from build123d import *

# Parameters (mm, degrees)
SKETCH1_W               = 24
SKETCH1_H               = 21
SKETCH1_R               = 1.625
BOSS_EXTRUDE1_DEPTH     = 8
BOSS_EXTRUDE4_DEPTH     = 45
CUT_EXTRUDE9_DEPTH      = 57.756194596
CUT_EXTRUDE9_DEPTH_BACK = 57.756194596
SKETCH15_R              = 1.75
FILLET3_R               = 2.5
SKETCH4_R               = 2.5625
CUT_EXTRUDE3_DEPTH      = 3
FILLET7_R               = 0.5
SKETCH20_R              = 2.75
CUT_EXTRUDE15_DEPTH     = 4
CUT_EXTRUDE16_DEPTH     = 4


with BuildPart() as part:
    # Sketch1 → Boss-Extrude1 (new body)
    with BuildSketch(Plane(origin=(0, 0, 0), x_dir=(1, 0, 0), z_dir=(0, 1, 0))):
        Rectangle(SKETCH1_W, SKETCH1_H)
        with Locations(Location((-9.5, 8, 0), (0, 0, 270))):
            Circle(SKETCH1_R, mode=Mode.SUBTRACT)
        with Locations(Location((9.5, 8, 0), (0, 0, 270))):
            Circle(SKETCH1_R, mode=Mode.SUBTRACT)
        with Locations(Location((9.5, -8, 0), (0, 0, 270))):
            Circle(SKETCH1_R, mode=Mode.SUBTRACT)
        with Locations(Location((-9.5, -8, 0), (0, 0, 270))):
            Circle(SKETCH1_R, mode=Mode.SUBTRACT)
    extrude(amount=BOSS_EXTRUDE1_DEPTH)

    # Sketch7 → Boss-Extrude4 (add)
    with BuildSketch(Plane(origin=(12, 0, 0), x_dir=(0, 0, -1), z_dir=(1, 0, 0))):
        Polygon((-20.5625, 21), (-20.5625, 8), (20.5625, 8), (20.5625, 21), (15.0625, 21), (15.0625, 11), (-15.0625, 11), (-15.0625, 21), align=None)
    extrude(amount=-BOSS_EXTRUDE4_DEPTH)

    # Sketch15 → Cut-Extrude9 (cut, two sides: drawn at the far end of the back side and taken through both)
    with BuildSketch(Plane.XY.offset(20.5625).offset(-CUT_EXTRUDE9_DEPTH_BACK)):
        with Locations((7, 16)):
            Circle(SKETCH15_R)
        with Locations((-10.5, 16)):
            Circle(SKETCH15_R)
        with Locations((-28, 16)):
            Circle(SKETCH15_R)
    extrude(amount=CUT_EXTRUDE9_DEPTH + CUT_EXTRUDE9_DEPTH_BACK, mode=Mode.SUBTRACT)

    # Fillet3
    fillet3_edges = [part.edges().sort_by_distance(p)[0] for p in [
        (0, 8, -10.5),
        (-10.5, 8, -20.5625),
        (-10.5, 8, 20.5625),
        (-10.5, 21, 20.5625),
        (-10.5, 21, -20.5625),
        (-12, 8, 0),
        (0, 8, 10.5),
    ]]
    fillet(fillet3_edges, radius=FILLET3_R)

    # Sketch4 → Cut-Extrude3 (cut)
    with BuildSketch(Plane(origin=(0, 11, 0), x_dir=(1, 0, 0), z_dir=(0, 1, 0))):
        with Locations(Location((-9.5, 8, 0), (0, 0, 270))):
            Circle(SKETCH4_R)
        with Locations((9.5, 8)):
            Circle(SKETCH4_R)
        with Locations((9.5, -8)):
            Circle(SKETCH4_R)
        with Locations(Location((-9.5, -8, 0), (0, 0, 270))):
            Circle(SKETCH4_R)
    extrude(amount=-CUT_EXTRUDE3_DEPTH, mode=Mode.SUBTRACT)

    # Fillet7
    fillet7_edges = [part.edges().sort_by_distance(p)[0] for p in [
        (12, 9.5, 8.5625),
        (12, 9.5, 7.4375),
        (12, 9.5, -7.4375),
        (12, 9.5, -8.5625),
    ]]
    fillet(fillet7_edges, radius=FILLET7_R)

    # Sketch20 → Cut-Extrude15 (cut)
    with BuildSketch(Plane.XY.offset(20.5625)):
        with Locations((-28, 16)):
            Circle(SKETCH20_R)
        with Locations((-10.5, 16)):
            Circle(SKETCH20_R)
        with Locations((7, 16)):
            Circle(SKETCH20_R)
    extrude(amount=-CUT_EXTRUDE15_DEPTH, mode=Mode.SUBTRACT)

    # Sketch21 → Cut-Extrude16 (cut)
    with BuildSketch(Plane(origin=(0, 0, -20.5625), x_dir=(-1, 0, 0), z_dir=(0, 0, -1))):
        Polygon((-5.441154273, 13.3), (-3.882308546, 16), (-5.441154273, 18.7), (-8.558845727, 18.7), (-10.117691454, 16), (-8.558845727, 13.3), align=None)
        Polygon((12.058845727, 13.3), (13.617691454, 16), (12.058845727, 18.7), (8.941154273, 18.7), (7.382308546, 16), (8.941154273, 13.3), align=None)
        Polygon((29.558845727, 13.3), (31.117691454, 16), (29.558845727, 18.7), (26.441154273, 18.7), (24.882308546, 16), (26.441154273, 13.3), align=None)
    extrude(amount=-CUT_EXTRUDE16_DEPTH, mode=Mode.SUBTRACT)


solid = part.part
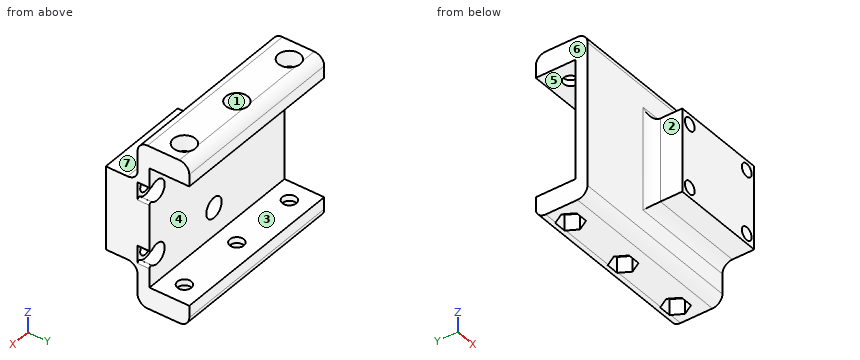
Verification items for the finished model (mm, model axes). Face numbers are marked on the shaded views. A direction names the side the tool comes from. Give positions to 0.01 mm unless a question says otherwise; leave off trailing zeros. Write each loop counter-clockwise with the first axis right and the second up, starting at its lowest first coordinate (ties: lowest second). Pieces come first, ordered by that corner, then holes. Notation, with made-up numbers: M -32,-5 L -11,-5 A21 cw -11,8 Z; hole C 76,59 d5. An arc over 180 degrees is marked long. Use CSV: the item, a comma, the result in double quotes.
1) Access from +Z, -Z, +X, -X, +Y, -Y to the whole of each face (thin tool, end or side, straight path). Record for the marked faces 1, 2 and 3.
Final values:
face 1,"+Z"
face 2,"+Z, -Z, -X, -Y"
face 3,"+X, -X, +Y"
2) Cross-section at D-D (x = -19.5). Enter the section's corners in (y, z).
Final values:
outline,"M 8,-18.06 A2.5 ccw 10.5,-20.56 L 18.5,-20.56 A2.5 ccw 21,-18.06 L 21,-15.06 L 11,-15.06 L 11,15.06 L 21,15.06 L 21,18.06 A2.5 ccw 18.5,20.56 L 10.5,20.56 A2.5 ccw 8,18.06 Z"
3) Release check for a two-part mould opening along Z. For the marked faces 4, 5, 6 and 7 record: released by +Z, released by -Z, zero draft, split by the parting line, or undercut.
Final values:
face 4,"undercut"
face 5,"undercut"
face 6,"zero draft"
face 7,"released by +Z"
4) Go/stop test with flat-tipped pins: pin 1 Ø3 at (x, z) = (-10, -11) entering from +Y; pin 2 Ø1 at (x, y) = (-4.5, 8) entering from +Z; pin 3 Ø3.5 at (x, z) = (9.5, 8) entering from -Y; pin 4 Ø2.5 at (x, z) = (-11, -17.5) entering from -Y. Record where each tip stops, or that it passes through.
Final values:
pin 1,"y = 11"
pin 2,"z = 19.56"
pin 3,"y = 0"
pin 4,"y = 8"
5) Cross-section at C-C (x = -28). Enter the section's corners in (y, z), plus the area to 3 significant figures.
Final values:
outline,"M 8,-18.06 A2.5 ccw 10.5,-20.56 L 13.3,-20.56 L 13.3,-16.56 L 14.25,-16.56 L 14.25,-15.06 L 11,-15.06 L 11,15.06 L 14.25,15.06 L 14.25,16.56 L 13.25,16.56 L 13.25,20.56 L 10.5,20.56 A2.5 ccw 8,18.06 Z; M 17.75,-16.56 L 18.7,-16.56 L 18.7,-20.55 A2.5 ccw 21,-18.06 L 21,-15.06 L 17.75,-15.06 Z; M 17.75,15.06 L 21,15.06 L 21,18.06 A2.5 ccw 18.75,20.55 L 18.75,16.56 L 17.75,16.56 Z"
area,"174 mm²"
6) Cross-section at B-B (y = 1.5). Enter the section's corners in (x, z) (3 decimals), plus the area to 3 significant figures.
Final values:
outline,"M -12,-10.5 L 12,-10.5 L 12,10.5 L -12,10.5 Z; hole C -9.5,-8 d3.25; hole C -9.5,8 d3.25; hole C 9.5,-8 d3.25; hole C 9.5,8 d3.25"
area,"471 mm²"
7) Material ranges on line 1 along X through (y, z) = (16, 15.5); line 2 along X through (y, z) = (2.25, -8) (3 decimals); line 3 along Z through (x, y) = (-18.5, 13), recorded low to high.
Final values:
line 1,"-33 to -29.75, -26.25 to -12.25, -8.75 to 5.25, 8.75 to 12"
line 2,"-12 to -11.125, -7.875 to 7.875, 11.125 to 12"
line 3,"-20.56 to -15.06, 15.06 to 20.56"
8) Cross-section at A-A (z = -7.5). Enter the section's corners in (x, y).
Final values:
outline,"M -33,8 L -14.5,8 A2.5 cw -12,5.5 L -12,0 L -11.05,0 L -11.05,8 L -12.01,8 L -12.01,11 L -33,11 Z; M -7.95,0 L 7.95,0 L 7.95,8 L 6.99,8 L 6.99,11 L -6.99,11 L -6.99,8 L -7.95,8 Z; M 11.05,0 L 12,0 L 12,8 L 11.05,8 Z"
